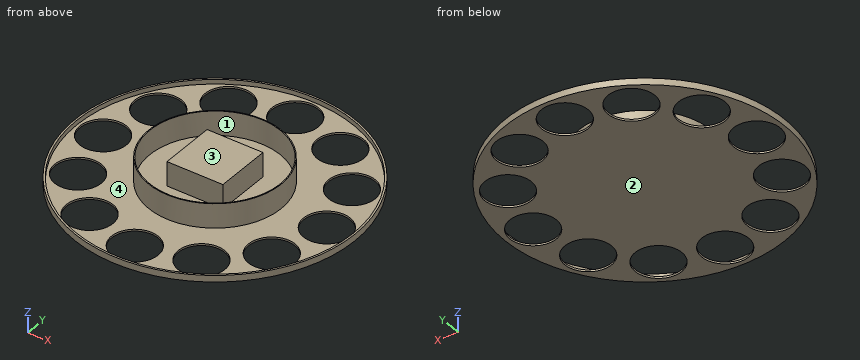
Autodesk Inventor part; units mm, degrees
ref_plane "YZ Plane" through (0, 0, 0) normal (1, 0, 0) x (0, 1, 0)
ref_plane "XZ Plane" through (0, 0, 0) normal (0, 1, 0) x (-1, 0, 0)
ref_plane "XY Plane" through (0, 0, 0) normal (0, 0, 1) x (1, 0, 0)
sketch "Sketch1" plane through (0, 0, 0) normal (0, 0, 1) x (1, 0, 0)
  circle A0 centre (0, 0) radius 150
  circle A1 centre (0, 120) radius 25
  circle A2 centre (60, 103.923) radius 25
  circle A3 centre (103.923, 60) radius 25
  circle A4 centre (120, 0) radius 25
  circle A5 centre (103.923, -60) radius 25
  circle A6 centre (60, -103.923) radius 25
  circle A7 centre (0, -120) radius 25
  circle A8 centre (-60, -103.923) radius 25
  circle A9 centre (-103.923, -60) radius 25
  circle A10 centre (-120, 0) radius 25
  circle A11 centre (-103.923, 60) radius 25
  circle A12 centre (-60, 103.923) radius 25
  dimension "d0" = 300
  dimension "d1" = 50
  dimension "d2" = 0
  dimension "d3" = 120
  dimension "d6" = 360
extrude "Extrusion1" add sketch "Sketch1" along normal blind 2
sketch "Sketch2" plane through (0, 0, 2) normal (0, 0, 1) x (1, 0, 0)
  circle A0 centre (0, 0) radius 150
  circle A1 centre (0, 0) radius 148
  dimension "d10" = 2
extrude "Extrusion2" add sketch "Sketch2" along normal blind 5
sketch "Sketch3" plane through (0, 0, 2) normal (0, 0, 1) x (1, 0, 0)
  circle A0 centre (0, 0) radius 71
  circle A1 centre (0, 0) radius 70
  line L0 (30, 30) -> (-30, 30)
  line L1 (-30, 30) -> (-30, -30)
  line L2 (-30, -30) -> (30, -30)
  line L3 (30, -30) -> (30, 30)
  line L4 (30, 30) -> (-30, -30) construction
  line L5 (-30, 30) -> (30, -30) construction
  dimension "d13" = 142
  dimension "d14" = 1
  dimension "d17" = 60
  dimension "d18" = 60
extrude "Extrusion3" add sketch "Sketch3" along normal blind 26
sketch "Sketch4" plane through (0, 0, 0) normal (0, 0, 1) x (1, 0, 0)
  point P0 (0, 0)
sketch "Sketch5" plane through (0, 0, 0) normal (0, 0, -1) x (-1, 0, 0)
  line L0 (-191.5583, 191.5583) -> (190.3872, 191.5583) construction
  line L1 (190.3872, 191.5583) -> (190.3872, -190.3872) construction
  line L2 (190.3872, -190.3872) -> (-191.5583, -190.3872) construction
  line L3 (-191.5583, -190.3872) -> (-191.5583, 191.5583) construction
  point P0 (0, 0)
properties part number "Clock"
Here's how the part is built. I have some questions about the finished solid (model axes, mm). Face numbers are marked on the shaded views. A direction names the side the tool comes from. Give positions to 0.01 mm unless a question says otherwise; leave off trailing zeros. Loops run counter-clockwise (first coordinate to the right, second up) from the corner with the lowest first, then second, coordinate; pieces in that order, holes last. Notation, with made-up numbers: (-15, 84) -> (42, 84) arc R10 ccw to (42, 101) -> close; hole circle Ø5 at (-31.5, 18). An arc over 180 degrees is marked (long way). Use one line per item in the form item = value. Start each with the question number.
1) Imagine slicing it at D-D (x = -61). Please give me the cut outline in (y, z).
2) For P1, Ø8, axis at x = 61.5, y = 53.5, coming from the +Z side; P2, Ø12, axis at y = 33, z = 15.5, coming from the -X side; P3, Ø2, axis at x = -46.5, z = 16.5, coming from the +Y side, each with a flat end and sliding along its axis, tell me the tip position at first contact or that it passes through.
3) Imagine slicing it at A-A (z = 23.75). Please give me the cut outline in (x, y), then the cut area to 3 significant figures.
4) Which directions (+Z, -Z, +X, -X, +Y, -Y) give clear straight access to the entire face, cutting with the end or side of a thin tool? Please do the marked faces 1 and 2.
5) Thinking about a two-plate mould opening in X: for the marked faces 3 and 4, which applies, +X half, -X half, draft (parallel to the pull), parting line (faces both ways), or undercut?
6) Imagine slicing it at B-B (x = 110). Please give me the cut outline in (y, z).
7) Imagine slicing it at C-C (y = -64). Please give me the cut outline in (x, z).
8) Please list where these lines run through material, in increasing order: line 1 along Y through (x, z) = (0, 0.65); line 2 along X through (y, z) = (4.5, 8.25); line 3 along Z through (x, y) = (30, 41.5).
Check values:
q1.outline = (-137.04, 0) -> (-128.9, 0) -> (-128.9, 2) -> (-134.84, 2) -> (-134.84, 7) -> (-137.04, 7) -> close; (-78.94, 0) -> (78.94, 0) -> (78.94, 2) -> (36.33, 2) -> (36.33, 28) -> (34.34, 28) -> (34.34, 2) -> (-34.34, 2) -> (-34.34, 28) -> (-36.33, 28) -> (-36.33, 2) -> (-78.94, 2) -> close; (128.9, 0) -> (137.04, 0) -> (137.04, 7) -> (134.84, 7) -> (134.84, 2) -> (128.9, 2) -> close
q2.P1 = 2
q2.P2 = -65.67
q2.P3 = 54.5
q3.outline = circle Ø142 at (0, 0); (-30, -30) -> (30, -30) -> (30, 30) -> (-30, 30) -> close; hole circle Ø140 at (0, 0)
q3.area = 4,040 mm^2
q4.face_1 = +Z
q4.face_2 = -Z, +X, -X, +Y, -Y
q5.face_3 = draft
q5.face_4 = undercut
q6.outline = (-101.98, 0) -> (-84.25, 0) -> (-84.25, 2) -> (-99.02, 2) -> (-99.02, 7) -> (-101.98, 7) -> close; (-35.75, 0) -> (-22.91, 0) -> (-22.91, 2) -> (-35.75, 2) -> close; (22.91, 0) -> (35.75, 0) -> (35.75, 2) -> (22.91, 2) -> close; (84.25, 0) -> (101.98, 0) -> (101.98, 7) -> (99.02, 7) -> (99.02, 2) -> (84.25, 2) -> close
q7.outline = (-135.66, 0) -> (-128.6, 0) -> (-128.6, 2) -> (-133.45, 2) -> (-133.45, 7) -> (-135.66, 7) -> close; (-79.25, 0) -> (79.25, 0) -> (79.25, 2) -> (30.74, 2) -> (30.74, 28) -> (28.35, 28) -> (28.35, 2) -> (-28.35, 2) -> (-28.35, 28) -> (-30.74, 28) -> (-30.74, 2) -> (-79.25, 2) -> close; (128.6, 0) -> (135.66, 0) -> (135.66, 7) -> (133.45, 7) -> (133.45, 2) -> (128.6, 2) -> close
q8.line_1 = -150 to -145, -95 to 95, 145 to 150
q8.line_2 = -70.86 to -69.86, -30 to 30, 69.86 to 70.86
q8.line_3 = 0 to 2
